Can you work these out from the model? Positions are in its coordinate system, mm. A direction names the side the tool comes from. Give positions to 0.01 mm unless a question says otherwise; leave off trailing zeros. Loops run counter-clockwise (first coordinate to the right, second up) from the corner with the lowest first, then second, coordinate; pieces in that order, holes last. Notation, with made-up numbers: (16, -32) - (52, -32) arc R28 ccw to (52, -2) - close; hole circle Ø3 at (50.5, 25). An arc over 180 degrees is marked (long way). Answer as a JSON object with one key per item and string values. Group by question number.
Item 1: Please list where these lines run through material, in increasing order: L1, parallel to Z at x = -7, y = -5.5; L2, parallel to X at y = -0.5, z = -84; L3, parallel to X at y = -3.25, z = -75.
Item 2: Suppose I cut it at B-B on z = -128. Write out the boundary of the cut face in (x, y).
Item 3: Suppose I cut it at D-D on x = 12. Write out the boundary of the cut face in (y, z), and give its area (3 significant figures).
Item 4: Which directions (+Z, -Z, +X, -X, +Y, -Y) give clear straight access to the entire face, cutting with the end or side of a thin tool? Please do faces 1 (the flat face through (6, 6, 0)), 2 (the flat face through (0, -12, 5)).
Item 5: Will these pins go through, and if not, where does the flat tip stop? pin 1 (8 mm diameter, centred on x = 2, z = -112, fed in from -Y); pin 2 (8 mm diameter, centred on y = -5, z = -127, fed in from +X); pin 3 (12 mm diameter, centred on x = -9, z = -56, fed in from +Y).
Solid Edge part; units mm, degrees
sketch "Sketch1" plane through (0, 0, 0) normal (0, 0, 1) x (1, 0, 0)
  circle A0 centre (0, 0) radius 13.92
extrude "Protrusion1" add sketch "Sketch1" along normal blind 10.32
sketch "Sketch2" plane through (0, 0, 0) normal (0, 0, -1) x (1, 0, 0)
  circle A0 centre (0, 0) radius 8
extrude "Protrusion2" add sketch "Sketch2" along normal blind 150
sketch "Sketch3" plane through (0, 0, -150) normal (0, 0, -1) x (1, 0, 0)
  circle A0 centre (0, 0) radius 7.9997
extrude "Cutout1" cut sketch "Sketch3" against normal blind 44 flip side to cut
chamfer "Chamfer_1" distance 1.2 angle 45 1 edges at (-7.9997, 0, -150)
sketch "Sketch4" plane through (0, 0, 10.32) normal (0, 0, 1) x (1, 0, 0)
  line L0 (-7.0545, 12) -> (7.0545, 12)
extrude "Cutout2" cut sketch "Sketch4" against normal up to next material side at (0, 12.05, 10.32)
pattern_circular "Pattern1" count 6 over 360 about axis through (0, 0, 10.32) along (0, 0, 1) of "Cutout2"
properties part number "215564" material "Stainless Steel, 304"
Worked out:
{
 "1": {"L1": "z = 0 to 10.32", "L2": "x = -7.98 to 7.98", "L3": "x = -7.31 to 7.31"},
 "2": {"outline": "circle Ø16 at (0, 0)"},
 "3": {"outline": "(-3.22, 0) - (3.22, 0) - (3.22, 10.32) - (-3.22, 10.32) - close", "area": "66.4 mm2"},
 "4": {"face 1": "-Z", "face 2": "+Z, -Z, +X, -X, -Y"},
 "5": {"pin 1": "stops at y = -8", "pin 2": "stops at x = 7.94", "pin 3": "stops at y = 7.42"}
}
